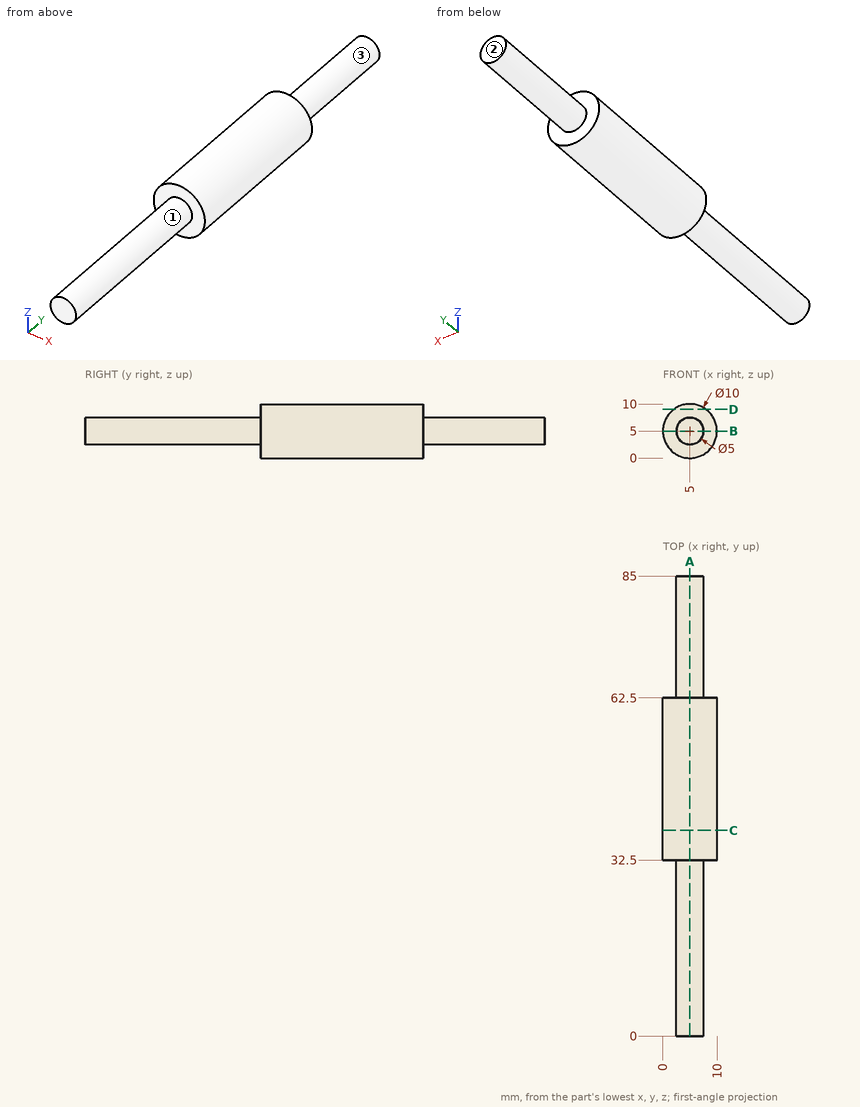
Job drawing, mm, ordinate dimensions from the low corner. One solid piece. A direction names the side the tool comes from. Give positions to 0.01 mm unless a question says otherwise; leave off trailing zeros. Order: outer loops, then holes, each group sorted by start corner. A loop starts at its lowest first (then second) coordinate and runs counter-clockwise, first axis right, second up. Notation, with made-up numbers: M 77.5,61 L 113.5,61 A20 ccw 113.5,68 Z; hole C -36.5,45 d2. An arc over 180 degrees is marked long. Put each result on its own line as item: value. Start each with the question number.
(1) Pin check, flat tips, straight feed: pin 1 Ø1.5 at (y, z) = (46, 3) entering from -X; pin 2 Ø6 at (x, z) = (2.5, 8.5) entering from +Y; pin 3 Ø1 at (y, z) = (56, 6) entering from +X; pin 4 Ø4 at (y, z) = (15, 5.5) entering from +X. Stop position of each tip, or through.
(2) Band-saw the part on B-B on z = 5. Give the cut face in (x, y).
(3) Drill centre lines: L1, parallel to X at y = 28.5, z = 5; L2, parallel to Y at x = 9.75, z = 6.25; L3, parallel to X at y = 26, z = 2.75. Where is each one in solid material? Low to high. Write a range as [from, to].
(4) Band-saw the part on C-C on y = 38. Give the cut face in (x, z).
(5) Tool access for the marked faces 1, 2 and 3: list every direction of +Z, -Z, +X, -X, +Y, -Y with a clear straight run to the whole face (end or side of a thin tool).
(6) Band-saw the part on D-D on z = 9. Give the cut face in (x, y), then the cut area to 3 significant figures.
(7) Band-saw the part on A-A on x = 5. Give the cut face in (y, z).
Results below:
1. pin 1: stops at x = 0.16
1. pin 2: stops at y = 85
1. pin 3: stops at x = 9.97
1. pin 4: stops at x = 7.5
2. outline: M 0,32.5 L 2.5,32.5 L 2.5,0 L 7.5,0 L 7.5,32.5 L 10,32.5 L 10,62.5 L 7.5,62.5 L 7.5,85 L 2.5,85 L 2.5,62.5 L 0,62.5 Z
3. L1: x = [2.5, 7.5]
3. L2: y = [32.5, 62.5]
3. L3: x = [3.91, 6.09]
4. outline: C 5,5 d10
5. face 1: -Y
5. face 2: +Z, -Z, +X, -X, +Y
5. face 3: +Y
6. outline: M 2,32.5 L 8,32.5 L 8,62.5 L 2,62.5 Z
6. area: 180 mm2
7. outline: M 0,2.5 L 32.5,2.5 L 32.5,0 L 62.5,0 L 62.5,2.5 L 85,2.5 L 85,7.5 L 62.5,7.5 L 62.5,10 L 32.5,10 L 32.5,7.5 L 0,7.5 Z
